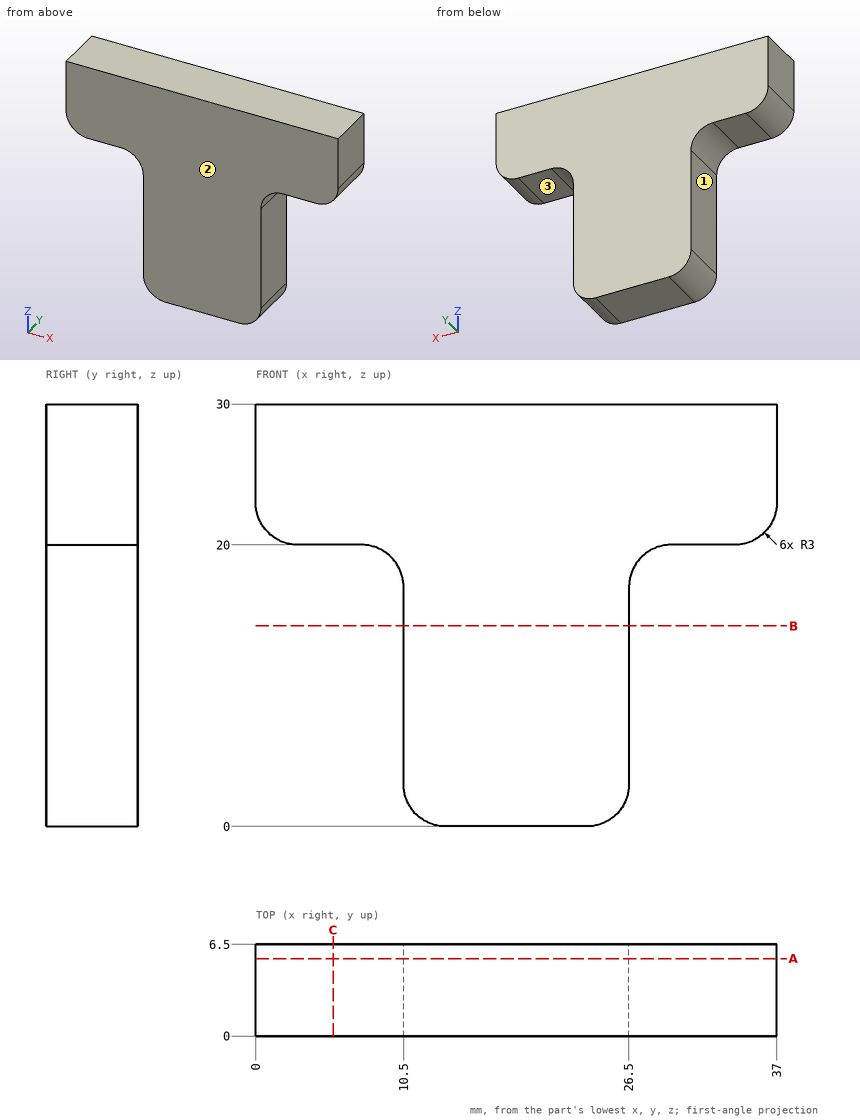
Verification items for this drawing (mm, ordinates from the low corner). A direction names the side the tool comes from. Coordinates: 2 decimals unless noted, no trailing zeros. Order: outer loops, then holes, each group sorted by start corner. A loop starts at its lowest first (then second) coordinate and runs counter-clockwise, first axis right, second up. Notation, with made-up numbers: M 64,52 L 109,52 A25 ccw 109,69 Z; hole C 20,47 d5. An arc over 180 degrees is marked long. One line per item, written item: value. Start each with the question number.
Item 1: Sectioned sample at B-B on z = 14.25. Record the cut outline in (x, y).
Item 2: Sectioned sample at A-A on y = 5.5. Record the cut outline in (x, z), then the cut area to 3 significant figures.
Item 3: Depth check by flat-ended pin: P1, Ø2, axis at y = 1, z = 17.5, coming from the +X side; P2, Ø2, axis at x = 31, y = 3.5, coming from the -Z side; P3, Ø3, axis at y = 4, z = 8.5, coming from the -X side. Enter the tip coordinate at first touch or a pass-through.
Item 4: Access from +Z, -Z, +X, -X, +Y, -Y to the whole of each face (thin tool, end or side, straight path). Record for the marked faces 1, 2 and 3.
Item 5: Thickness scan on probe 1 along X at (y, z) = (6, 13); probe 2 along Z at (x, y) = (32, 5.5); probe 3 along Z at (x, y) = (2, 1.75). Record the ranges inside material, lowest first.
Item 6: Sectioned sample at C-C on x = 5.5. Record the cut outline in (y, z).
Calculated:
1. outline: M 10.5,0 L 26.5,0 L 26.5,6.5 L 10.5,6.5 Z
2. outline: M 0,23 A3 ccw 3,20 L 7.5,20 A3 cw 10.5,17 L 10.5,3 A3 ccw 13.5,0 L 23.5,0 A3 ccw 26.5,3 L 26.5,17 A3 cw 29.5,20 L 34,20 A3 ccw 37,23 L 37,30 L 0,30 Z
2. area: 686 mm^2
3. P1: x = 26.9
3. P2: z = 20
3. P3: x = 10.5
4. face 1: -Z, -X, +Y, -Y
4. face 2: +Z, -Z, +X, -X, -Y
4. face 3: -Z, +X, +Y, -Y
5. probe 1: 10.5 to 26.5
5. probe 2: 20 to 30
5. probe 3: 20.17 to 30
6. outline: M 0,20 L 6.5,20 L 6.5,30 L 0,30 Z
